Input: dimensioned drawing with shaded views. Units: mm. Origin: part minimum x, y, z. A direction names the side the tool comes from. Give positions to 0.01 mm unless a question says otherwise; leave off trailing zeros. Loops run counter-clockwise (first coordinate to the right, second up) from the corner with the lowest first, then second, coordinate; pieces in that order, holes last. Notation, with made-up numbers: M -23.5,16.25 L 12.5,16.25 A18 ccw 12.5,39.25 Z; hole C -28,8 d2. An arc over 180 degrees is marked long. Answer in a Markdown table with one row per item.
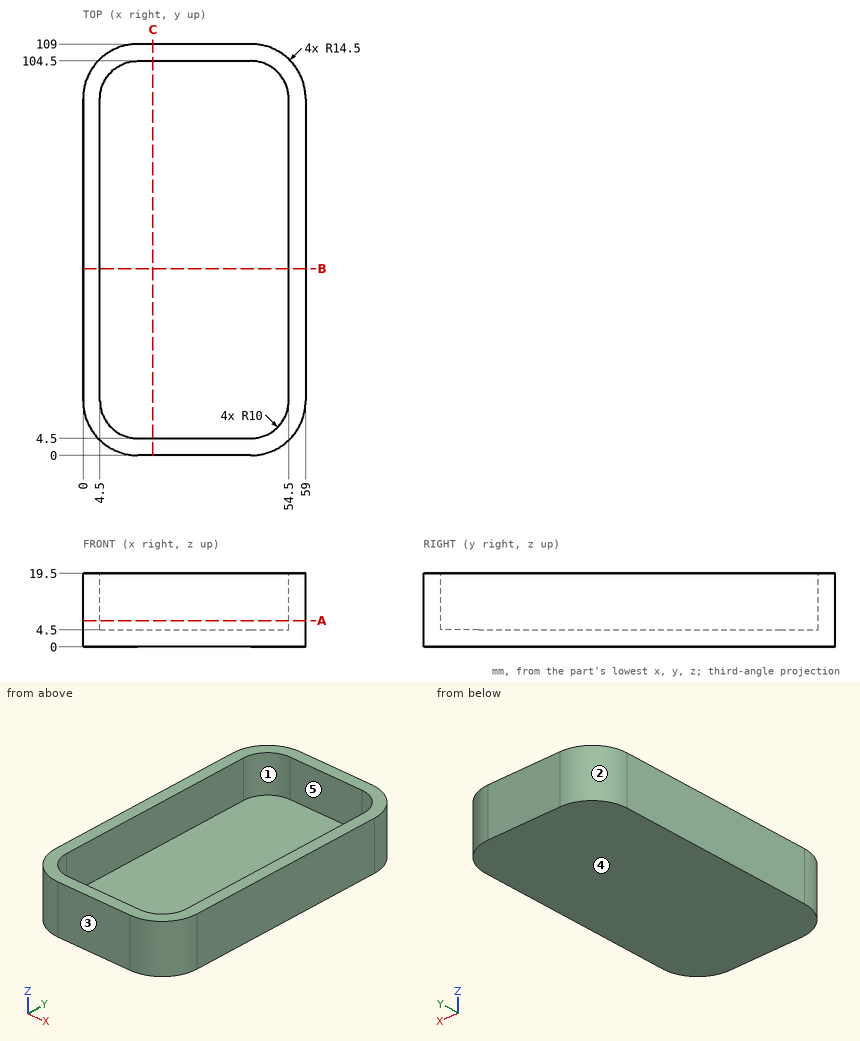
Q1. Reachability of the marked faces 4 and 5 from +Z, -Z, +X, -X, +Y, -Y: full face, straight path, thin tool, end or side. Return the list, or none.
Values follow:
| item | result |
|---|---|
| face 4 | -Z, +X, -X, +Y, -Y |
| face 5 | +Z |
Q2. Ray query, probe 1 along Y at (x, z) = (33, 7); probe 2 along X at (y, z) = (71, 8.75); probe 3 along Z at (x, y) = (6, 56). Return the intervals inside material, ascending. Write a range as from..to.
Values follow:
| item | result |
|---|---|
| probe 1 | 0..4.5, 104.5..109 |
| probe 2 | 0..4.5, 54.5..59 |
| probe 3 | 0..4.5 |
Q3. Section query A-A (z = 7). Output: boundary loops of the cut face in (x, y), plus the area to 3 significant figures.
Values follow:
| item | result |
|---|---|
| outline | M 0,14.5 A14.5 ccw 14.5,0 L 44.5,0 A14.5 ccw 59,14.5 L 59,94.5 A14.5 ccw 44.5,109 L 14.5,109 A14.5 ccw 0,94.5 Z; hole M 4.5,14.5 A10 ccw 14.5,4.5 L 44.5,4.5 A10 ccw 54.5,14.5 L 54.5,94.5 A10 ccw 44.5,104.5 L 14.5,104.5 A10 ccw 4.5,94.5 Z |
| area | 1,340 mm^2 |
Q4. Section query C-C (x = 18.5). Output: boundary loops of the cut face in (y, z), plus the area to 4 significant figures.
Values follow:
| item | result |
|---|---|
| outline | M 0,0 L 109,0 L 109,19.5 L 104.5,19.5 L 104.5,4.5 L 4.5,4.5 L 4.5,19.5 L 0,19.5 Z |
| area | 625.5 mm^2 |
Q5. Contact query for a flat-ended pin moving along its axis: pin 1 Ø12 at (x, y) = (31.5, 75) entering from +Z. Output: stop coordinate, or through.
Values follow:
| item | result |
|---|---|
| pin 1 | z = 4.5 |
Q6. Section query B-B (y = 49.5). Output: boundary loops of the cut face in (x, z), plus the area to 4 significant figures.
Values follow:
| item | result |
|---|---|
| outline | M 0,0 L 59,0 L 59,19.5 L 54.5,19.5 L 54.5,4.5 L 4.5,4.5 L 4.5,19.5 L 0,19.5 Z |
| area | 400.5 mm^2 |
Q7. Mould query, pull axis X, two halves, no side actions, for the marked faces 1, 2 and 3. Classes: +X half, -X half, draft (parallel to the pull), parting line (faces both ways), or undercut.
Values follow:
| item | result |
|---|---|
| face 1 | undercut |
| face 2 | -X half |
| face 3 | draft |
